Autodesk Inventor part; units mm, degrees
ref_plane "YZ Plane" through (0, 0, 0) normal (1, 0, 0) x (0, 1, 0)
ref_plane "XZ Plane" through (0, 0, 0) normal (0, 1, 0) x (-1, 0, 0)
ref_plane "XY Plane" through (0, 0, 0) normal (0, 0, 1) x (1, 0, 0)
sketch "Sketch1" plane through (0, 0, 0) normal (0, 1, 0) x (-1, 0, 0)
  point P0 (0, 0)
sketch "Sketch2" plane through (0, 0, 0) normal (0, 1, 0) x (-1, 0, 0)
  circle A0 centre (0, 0) radius 11
  circle A1 centre (0, 0) radius 14
  dimension "d0" = 22
  dimension "d1" = 28
extrude "Extrusion1" add sketch "Sketch2" along normal blind 90 contours A0 | A1
hole "Hole1" at (0, 90, 0) direction (0, -1, 0) diameter 22 depth 90 tip angle 118
sketch "Sketch3" plane through (0, 90, 0) normal (0, 1, 0) x (1, 0, 0)
  circle A0 centre (0, 0) radius 11
  circle A1 centre (0, 0) radius 14
  line L0 (2.5, 13.775) -> (2.5, 10.7121)
  line L1 (-2.5, 13.775) -> (-2.5, 10.7121)
  line L2 (-2.5, -10.7121) -> (-2.5, -13.775)
  line L3 (2.5, -10.7121) -> (2.5, -13.775)
extrude "Extrusion2" cut sketch "Sketch3" against normal blind 5 contours L3 A1 L2 A0
sketch "Sketch4" plane through (0, 90, 0) normal (0, 1, 0) x (1, 0, 0)
  arc A0 (2.5, -10.7121) -> (-2.5, -10.7121) centre (0, 0) ccw
  circle A1 centre (0, 0) radius 14
  line L0 (-2.5, 13.775) -> (-2.5, 10.7121)
  circle A2 centre (0, 0) radius 11
  line L1 (2.5, 13.775) -> (2.5, 10.7121)
sketch "Sketch5" plane through (0, 90, 0) normal (0, 1, 0) x (1, 0, 0)
  point P0 (0, 0)
sketch "Sketch6" plane through (0, 90, 0) normal (0, 1, 0) x (1, 0, 0)
  point P0 (0, 0)
extrude "Extrusion3" cut sketch "Sketch4" against normal blind 5 contours A0 L0 A1 L1
sketch "Sketch7" plane through (0, 90, 0) normal (0, 1, 0) x (1, 0, 0)
  point P0 (0, 0)
  point P1 (-2.4887, 10.7148)
  point P2 (2.5, 10.7121)
sketch "Sketch8" plane through (0, 0, 0) normal (0, 1, 0) x (-1, 0, 0)
  arc A0 (2.5, -10.7121) -> (-2.5, -10.7121) centre (0, 0) ccw
sketch "Sketch9" plane through (0, 85, 0) normal (0, 1, 0) x (1, 0, 0)
  arc A0 (-2.5, 13.775) -> (-2.5, -13.775) centre (0, 0) ccw
  line L0 (-14, 0) -> (14.5387, 0)
properties part number "pusher"
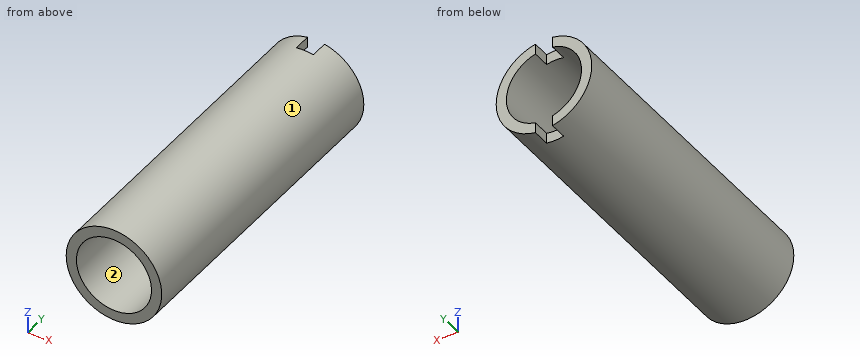
The model under review builds one solid part; all positions refer to its coordinate system, in mm. Face numbers are marked on the shaded views. Give positions to 0.01 mm unless a question says otherwise; leave off trailing zeros. Loops run counter-clockwise (first coordinate to the right, second up) from the corner with the lowest first, then second, coordinate; pieces in that order, holes last. Notation, with made-up numbers: (-38, 0.25) -> (5, 0.25) arc R19 ccw to (5, 5.25) -> close; hole circle Ø5 at (-25, 48.25). An arc over 180 degrees is marked (long way). Use CSV: the item, a comma, the result in double quotes.
1. Consider section C-C, the plane y = 25. Write out the cut boundary in (x, z).
Result:
outline,"circle Ø28 at (0, 0); hole circle Ø22 at (0, 0)"
2. To check wall thickness, follow probe 1 along X at (y, z) = (62, 0); probe 2 along X at (y, z) = (61, 4). State the ranges of each line that lie inside material, in increasing order. Write a range as from..to.
Result:
probe 1,"x = -14..-11, 11..14"
probe 2,"x = -13.42..-10.25, 10.25..13.42"
3. For P1, Ø4, axis at y = 27.5, z = 7.5, coming from the +X side; P2, Ø0.9, axis at y = 87.5, z = 12, coming from the -X side; P3, Ø12, axis at x = -8, y = 77.5, coming from the -Z side, all flat-tipped, find the tip position at first contact; note any pin that passes through.
Result:
P1,"stops at x = 12.87"
P2,"stops at x = -7.91"
P3,"stops at z = -13.86"
4. Consider section B-B, the plane x = 0. Write out the cut boundary in (y, z), then the cut area to 3 significant figures.
Result:
outline,"(0, -14) -> (85, -14) -> (85, -11) -> (0, -11) -> close; (0, 11) -> (85, 11) -> (85, 14) -> (0, 14) -> close"
area,"510 mm²"
5. Consider section A-A, the plane z = 0. Write out the cut boundary in (x, y), then the cut area to 3 significant figures.
Result:
outline,"(-14, 0) -> (-11, 0) -> (-11, 90) -> (-14, 90) -> close; (11, 0) -> (14, 0) -> (14, 90) -> (11, 90) -> close"
area,"540 mm²"
6. The part is to be moulded in two halves that separate along Z. For the marked faces 1 and 2, say which applies: +Z half, -Z half, draft (parallel to the pull), parting line (faces both ways), or undercut.
Result:
face 1,"parting line"
face 2,"undercut"
